```python
from build123d import *

# Parameters (mm, degrees)
SKETCH_1_R      = 2
SKETCH_1_R_2    = 1.7
SKETCH_1_R_3    = 1.5
SKETCH_1_R_4    = 3.25
EXTRUDE_1_DEPTH = 1.5


with BuildPart() as part:
    # 草图1 → 凸台-拉伸1 (new body)
    with BuildSketch(Plane(origin=(0, 0, 0), x_dir=(1, 0, 0), z_dir=(0, 1, 0))):
        with BuildLine():
            Line((19.75, 2.165063509), (5.096488448, 10.625272348))
            ThreePointArc((5.096488448, 10.625272348), (4.922427124, 10.704637858), (4.736437674, 10.749405626))
            Line((4.736437674, 10.749405626), (-2.101908222, 11.7159388))
            ThreePointArc((-2.101908222, 11.7159388), (-4.61878361, 14.995906411), (-6.744553684, 11.449929699))
            ThreePointArc((-6.744553684, 11.449929699), (-6.675732942, 10.813623622), (-7.006838923, 10.265909693))
            Line((-7.006838923, 10.265909693), (-14.905573539, 3.595069524))
            ThreePointArc((-14.905573539, 3.595069524), (-15.456234647, 3.363542696), (-16.040639512, 3.487249128))
            ThreePointArc((-16.040639512, 3.487249128), (-22, 0), (-16.040639512, -3.487249128))
            ThreePointArc((-16.040639512, -3.487249128), (-15.456234647, -3.363542696), (-14.905573539, -3.595069524))
            Line((-14.905573539, -3.595069524), (-7.006838923, -10.265909693))
            ThreePointArc((-7.006838923, -10.265909693), (-6.675732942, -10.813623622), (-6.744553684, -11.449929699))
            ThreePointArc((-6.744553684, -11.449929699), (-4.61878361, -14.995906411), (-2.101908222, -11.7159388))
            Line((-2.101908222, -11.7159388), (4.736437674, -10.749405626))
            ThreePointArc((4.736437674, -10.749405626), (4.922427124, -10.704637858), (5.096488448, -10.625272348))
            Line((5.096488448, -10.625272348), (19.75, -2.165063509))
            ThreePointArc((19.75, -2.165063509), (20.25, -2.031088913), (20.75, -2.165063509))
            ThreePointArc((20.75, -2.165063509), (24.5, 0), (20.75, 2.165063509))
            ThreePointArc((20.75, 2.165063509), (20.25, 2.031088913), (19.75, 2.165063509))
        make_face()
        Circle(SKETCH_1_R, mode=Mode.SUBTRACT)
        with Locations((-18, 0)):
            Circle(SKETCH_1_R_2, mode=Mode.SUBTRACT)
        with Locations((22, 0)):
            Circle(SKETCH_1_R_3, mode=Mode.SUBTRACT)
        with Locations((-4.47577596, 12.5)):
            Circle(SKETCH_1_R_3, mode=Mode.SUBTRACT)
        with Locations((-4.47577596, -12.5)):
            Circle(SKETCH_1_R_3, mode=Mode.SUBTRACT)
        with Locations((15.2, 0)):
            Circle(SKETCH_1_R_4, mode=Mode.SUBTRACT)
        with BuildLine():
            Line((2.23143448, 9.588554578), (-1.256530939, 10.081544307))
            ThreePointArc((-1.256530939, 10.081544307), (-2.171731289, 9.72303877), (-2.33794765, 8.754281823))
            Line((-2.33794765, 8.754281823), (-0.872808817, 4.662424773))
            ThreePointArc((-0.872808817, 4.662424773), (-0.512657064, 4.185850496), (0.054926934, 3.999622861))
            ThreePointArc((0.054926934, 3.999622861), (0.187612888, 3.995597753), (0.320092213, 3.987172052))
            ThreePointArc((0.320092213, 3.987172052), (0.902629068, 4.119395878), (1.305852753, 4.56012594))
            Line((1.305852753, 4.56012594), (2.997222742, 8.174556771))
            ThreePointArc((2.997222742, 8.174556771), (2.970810351, 9.074617878), (2.23143448, 9.588554578))
        make_face(mode=Mode.SUBTRACT)
        with BuildLine():
            Line((12.853062501, 4.414961424), (5.956182941, 8.396876694))
            ThreePointArc((5.956182941, 8.396876694), (5.156119776, 8.484770625), (4.550445454, 7.954690416))
            Line((4.550445454, 7.954690416), (2.664458984, 3.924367251))
            ThreePointArc((2.664458984, 3.924367251), (2.584431714, 3.332397688), (2.856157177, 2.800422501))
            ThreePointArc((2.856157177, 2.800422501), (4, 0), (2.856157177, -2.800422501))
            ThreePointArc((2.856157177, -2.800422501), (2.584431714, -3.332397688), (2.664458984, -3.924367251))
            Line((2.664458984, -3.924367251), (4.550445454, -7.954690416))
            ThreePointArc((4.550445454, -7.954690416), (4.374221674, -8.659373504), (4.721405489, -9.297414626))
            Line((4.721405489, -9.297414626), (13.026112738, -4.50268966))
            ThreePointArc((13.026112738, -4.50268966), (10.200941154, -0.097008541), (12.853062501, 4.414961424))
        make_face(mode=Mode.SUBTRACT)
        with BuildLine():
            Line((-2.33794765, -8.754281823), (-0.872808817, -4.662424773))
            ThreePointArc((-0.872808817, -4.662424773), (-0.512657064, -4.185850496), (0.054926934, -3.999622861))
            ThreePointArc((0.054926934, -3.999622861), (0.187612888, -3.995597753), (0.320092213, -3.987172052))
            ThreePointArc((0.320092213, -3.987172052), (0.902629068, -4.119395878), (1.305852753, -4.56012594))
            Line((1.305852753, -4.56012594), (2.997222742, -8.174556771))
            ThreePointArc((2.997222742, -8.174556771), (2.970810351, -9.074617878), (2.23143448, -9.588554578))
            Line((2.23143448, -9.588554578), (-1.256530939, -10.081544307))
            ThreePointArc((-1.256530939, -10.081544307), (-2.171731289, -9.72303877), (-2.33794765, -8.754281823))
        make_face(mode=Mode.SUBTRACT)
        with BuildLine():
            Line((-5.622052564, 9.472053038), (-13.937734763, 2.449081695))
            ThreePointArc((-13.937734763, 2.449081695), (-14.258158429, 1.944937864), (-14.23400713, 1.348071847))
            ThreePointArc((-14.23400713, 1.348071847), (-14, 0), (-14.23400713, -1.348071847))
            ThreePointArc((-14.23400713, -1.348071847), (-14.258158429, -1.944937864), (-13.937734763, -2.449081695))
            Line((-13.937734763, -2.449081695), (-5.622052564, -9.472053038))
            ThreePointArc((-5.622052564, -9.472053038), (-4.717022681, -9.673722513), (-4.035359228, -9.045164955))
            Line((-4.035359228, -9.045164955), (-2.285010045, -4.156769069))
            ThreePointArc((-2.285010045, -4.156769069), (-2.260804326, -3.559905256), (-2.581182025, -3.055732213))
            ThreePointArc((-2.581182025, -3.055732213), (-4, 0), (-2.581182025, 3.055732213))
            ThreePointArc((-2.581182025, 3.055732213), (-2.260804326, 3.559905256), (-2.285010045, 4.156769069))
            Line((-2.285010045, 4.156769069), (-4.035359228, 9.045164955))
            ThreePointArc((-4.035359228, 9.045164955), (-4.717022681, 9.673722513), (-5.622052564, 9.472053038))
        make_face(mode=Mode.SUBTRACT)
    extrude(amount=EXTRUDE_1_DEPTH)


solid = part.part
```
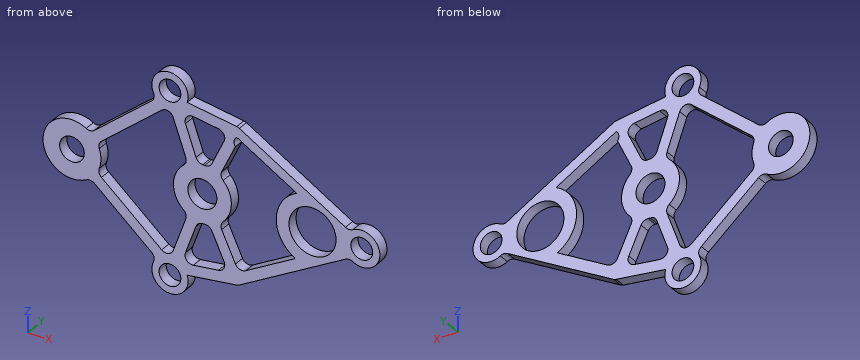
Check sheet for the modelled part. Datum: model origin and axes. Units: mm. Coordinates: 2 decimals unless noted, no trailing zeros. Write each loop counter-clockwise with the first axis right and the second up, starting at its lowest first coordinate (ties: lowest second). Pieces come first, ordered by that corner, then holes. Notation, with made-up numbers: (-36, 77) -> (19, 77) arc R8 cw to (19, 85) -> close; hole circle Ø1 at (80.25, 84). An arc over 180 degrees is marked (long way). Use a Markdown table: item, result.
1. Sectioned sample at B-B (z = 12.5). Enter the section's corners in (x, y).
Reported:
| item | result |
|---|---|
| outline | (-6.98, 0) -> (-5.98, 0) -> (-5.98, 1.5) -> (-6.98, 1.5) -> close; (-2.98, 0) -> (-1.98, 0) -> (-1.98, 1.5) -> (-2.98, 1.5) -> close |
2. Sectioned sample at A-A (x = 22). Enter the section's corners in (y, z), plus the area to 3 significant figures.
Reported:
| item | result |
|---|---|
| outline | (0, -2.5) -> (1.5, -2.5) -> (1.5, -1.5) -> (0, -1.5) -> close; (0, 1.5) -> (1.5, 1.5) -> (1.5, 2.5) -> (0, 2.5) -> close |
| area | 3.00 mm2 |
3. Sectioned sample at D-D (y = 0.7). Give the number of separate pieces and of enclosed holes in the cut face, plus the area to 3 significant figures.
Reported:
| item | result |
|---|---|
| separate pieces | 1 |
| enclosed holes | 10 |
| area | 286 mm2 |
4. Sectioned sample at C-C (z = -5.5). Enter the section's corners in (x, y), plus the area to 3 significant figures.
Reported:
| item | result |
|---|---|
| outline | (-12.65, 0) -> (-10.33, 0) -> (-10.33, 1.5) -> (-12.65, 1.5) -> close; (-2.77, 0) -> (-1.17, 0) -> (-1.17, 1.5) -> (-2.77, 1.5) -> close; (1.75, 0) -> (3.4, 0) -> (3.4, 1.5) -> (1.75, 1.5) -> close; (10.97, 0) -> (13.97, 0) -> (13.97, 1.5) -> (10.97, 1.5) -> close |
| area | 12.9 mm2 |
5. Scan lines: line 1 along X through (y, z) = (0.3, 6) (3 decimals); line 2 along X through (y, z) = (0.3, -12.5); line 3 along X through (y, z) = (0.35, 9). Record each from-to range of solid material in increasing order.
Reported:
| item | result |
|---|---|
| line 1 | x = -12.058 to -9.733, -2.945 to -1.352, 1.98 to 3.636, 10.433 to 13.108 |
| line 2 | x = -6.98 to -5.98, -2.98 to -1.98 |
| line 3 | x = -8.51 to -6.18, -4.02 to -2.39, 3.01 to 4.48, 5.24 to 7.91 |
